Check sheet for the modelled part. Datum: model origin and axes. Units: mm. Face numbers are marked on the shaded views. A direction names the side the tool comes from. Round coordinates to 2 decimals unless told otherwise and drop trailing zeros. Write each loop counter-clockwise with the first axis right and the second up, starting at its lowest first coordinate (ties: lowest second). Pieces come first, ordered by that corner, then holes. Notation, with made-up numbers: M 1.25,20 L 52.25,20 A30 cw 52.25,57 Z; hole C 47,71 d11. An arc over 180 degrees is marked long. Answer in a Markdown table with one row per item.
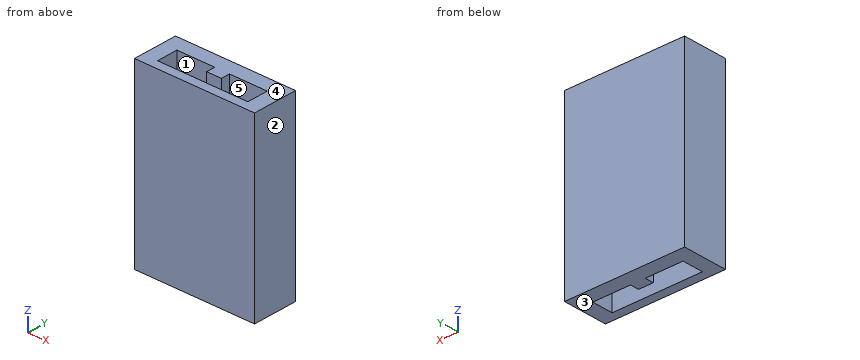
Autodesk Inventor part; units mm, degrees
ref_plane "YZ Plane" through (0, 0, 0) normal (1, 0, 0) x (0, 1, 0)
ref_plane "XZ Plane" through (0, 0, 0) normal (0, 1, 0) x (-1, 0, 0)
ref_plane "XY Plane" through (0, 0, 0) normal (0, 0, 1) x (1, 0, 0)
sketch "スケッチ1" plane through (0, 0, 0) normal (0, 1, 0) x (-1, 0, 0)
  line L0 (0, 0) -> (40, 0)
  line L1 (40, 0) -> (40, -60)
  line L2 (40, -60) -> (0, -60)
  line L3 (0, -60) -> (0, 0)
  dimension "d0" = 40
  dimension "d1" = 60
extrude "押し出し1" add sketch "スケッチ1" along normal blind 15
ref_plane "作業平面1" through (-40, 0, 0) normal (0, 0, 1) x (1, 0, 0)
sketch "スケッチ2" plane through (-40, 0, 0) normal (0, 0, 1) x (1, 0, 0)
  line L0 (40, 15) -> (0, 15)
  line L1 (0, 0) -> (40, 0)
  line L2 (0, 0) -> (0, 15)
  line L3 (40, 0) -> (40, 15)
  line L4 (4.95, 3) -> (35.05, 3)
  line L5 (35.05, 3) -> (35.05, 10.1)
  line L6 (35.05, 10.1) -> (4.95, 10.1)
  line L7 (4.95, 10.1) -> (4.95, 3)
  point P0 (20, 10.1)
  dimension "d6" = 15
  dimension "d7" = 40
  dimension "d8" = 30.1
  dimension "d9" = 7.1
  dimension "d10" = 3
extrude "押し出し2" cut sketch "スケッチ2" against normal through all contours L7 L6 L5 L4
ref_plane "作業平面2" through (-35.05, 10.1, -60) normal (0, -1, 0) x (1, 0, 0)
sketch "スケッチ3" plane through (-35.05, 10.1, -60) normal (0, -1, 0) x (1, 0, 0)
  line L0 (-4.95, 60) -> (35.05, 60)
  line L1 (12.6, 60) -> (17.5, 60)
  line L2 (17.5, 60) -> (17.5, 0)
  line L3 (17.5, 0) -> (12.6, 0)
  line L4 (12.6, 0) -> (12.6, 60)
  point P0 (15.05, 60)
  dimension "d15" = 60
  dimension "d16" = 4.9
extrude "押し出し3" add sketch "スケッチ3" along normal blind 2.95
properties part number "linia"
1. Access from +Z, -Z, +X, -X, +Y, -Y to the whole of each face (thin tool, end or side, straight path). Record for the marked faces 4 and 5.
Found:
| item | result |
|---|---|
| face 4 | +Z, +X, -X, +Y, -Y |
| face 5 | +Z, -Z |
2. Scan lines: L1, parallel to X at y = 8.5, z = -24; L2, parallel to X at y = 6, z = -40; L3, parallel to Y at x = -21, z = -6.5. Record each from-to range of solid material in increasing order.
Found:
| item | result |
|---|---|
| L1 | x = -40 to -35.05, -22.45 to -17.55, -4.95 to 0 |
| L2 | x = -40 to -35.05, -4.95 to 0 |
| L3 | y = 0 to 3, 7.15 to 15 |
3. Section check B-B, the plane y = 8.5. Record the cut outline in (x, z).
Found:
| item | result |
|---|---|
| outline | M -40,-60 L -35.05,-60 L -35.05,0 L -40,0 Z; M -22.45,-60 L -17.55,-60 L -17.55,0 L -22.45,0 Z; M -4.95,-60 L 0,-60 L 0,0 L -4.95,0 Z |
4. Section check D-D, the plane y = 3.75. Record the cut outline in (x, z), and give its area (3 significant figures).
Found:
| item | result |
|---|---|
| outline | M -40,-60 L -35.05,-60 L -35.05,0 L -40,0 Z; M -4.95,-60 L 0,-60 L 0,0 L -4.95,0 Z |
| area | 594 mm2 |
5. Section check C-C, the plane x = -9. Record the cut outline in (y, z).
Found:
| item | result |
|---|---|
| outline | M 0,-60 L 3,-60 L 3,0 L 0,0 Z; M 10.1,-60 L 15,-60 L 15,0 L 10.1,0 Z |
6. Draft check along X on the marked faces 1, 2 and 3. Enter one of: +X half, -X half, draft (parallel to the pull), parting line (faces both ways), or undercut.
Found:
| item | result |
|---|---|
| face 1 | undercut |
| face 2 | +X half |
| face 3 | draft |
7. Section check A-A, the plane z = -38.5. Record the cut outline in (x, y).
Found:
| item | result |
|---|---|
| outline | M -40,0 L 0,0 L 0,15 L -40,15 Z; hole M -35.05,3 L -4.95,3 L -4.95,10.1 L -17.55,10.1 L -17.55,7.15 L -22.45,7.15 L -22.45,10.1 L -35.05,10.1 Z |
